from build123d import *

# Parameters (mm, degrees)
CROQUIS1_W              = 460
CROQUIS1_H              = 660
SALIENTE_EXTRUIR1_DEPTH = 10
VACIADO1_T              = -2


with BuildPart() as part:
    # Croquis1 → Saliente-Extruir1 (new body)
    with BuildSketch(Plane.XY):
        Rectangle(CROQUIS1_W, CROQUIS1_H)
    extrude(amount=SALIENTE_EXTRUIR1_DEPTH)

    # Vaciado1
    vaciado1_openings = [part.faces().sort_by_distance(p)[0] for p in [
        (0, 0, 0),
    ]]
    offset(amount=VACIADO1_T, openings=vaciado1_openings, kind=Kind.INTERSECTION)


solid = part.part
Could you check a few things on this model? Use its own coordinates, in mm. Give positions to 0.01 mm unless a question says otherwise; leave off trailing zeros. Order: outer loops, then holes, each group sorted by start corner. A loop starts at its lowest first (then second) coordinate and runs counter-clockwise, first axis right, second up. Notation, with made-up numbers: (15, -28) - (50, -28) arc R15 cw to (50, -16) - close; hole circle Ø6 at (41.25, -35). An arc over 180 degrees is marked (long way). Return JSON: item names as keys, results as strings. Group by question number.
Q1. Thinking about a two-plate mould opening in Y: for faces 1 (the face through (-3, 5, 8)), 2 (the face through (-3, 5, 10)), which applies, pulls with the +Y half, pulls with the -Y half, needs draft (parallel to the pull), parting line crosses it, or undercut?
Q2. Will this pin go through, and if not, where does the flat tip stop? pin 1 Ø1 at (x, y) = (99, 216.5) entering from -Z.
Q3. Suppose I cut it at A-A, the plane z = 1.5. Please give me the cut outline in (x, y), and give its area (3 significant figures).
Q4. Please list where these lines run through material, in increasing order: line 1 along X through (y, z) = (251.5, 2); line 2 along Y through (x, z) = (123, 5); line 3 along Z through (x, y) = (92, 231). Write a range as [from, to].
Q5. Suppose I cut it at C-C, the plane y = -214. Please give me the cut outline in (x, z).
Q6. Suppose I cut it at B-B, the plane x = -131. Please give me the cut outline in (y, z).
Resolved:
{
 "1": {"face 1": "undercut", "face 2": "needs draft"},
 "2": {"pin 1": "stops at z = 8"},
 "3": {"outline": "(-230, -330) - (230, -330) - (230, 330) - (-230, 330) - close; hole (-228, -328) - (228, -328) - (228, 328) - (-228, 328) - close", "area": "4,460 mm2"},
 "4": {"line 1": "x = [-230, -228], [228, 230]", "line 2": "y = [-330, -328], [328, 330]", "line 3": "z = [8, 10]"},
 "5": {"outline": "(-230, 0) - (-228, 0) - (-228, 8) - (228, 8) - (228, 0) - (230, 0) - (230, 10) - (-230, 10) - close"},
 "6": {"outline": "(-330, 0) - (-328, 0) - (-328, 8) - (328, 8) - (328, 0) - (330, 0) - (330, 10) - (-330, 10) - close"}
}
